CAD build for the part. Positions are in the model's coordinates, mm. A direction names the side the tool comes from. Give positions to 0.01 mm unless a question says otherwise; leave off trailing zeros. Order: outer loops, then holes, each group sorted by start corner. A loop starts at its lowest first (then second) coordinate and runs counter-clockwise, first axis right, second up.
Item 1: Band-saw the part on A-A on z = 86. Give the cut face in (x, y).
Item 2: Which spindle directions (+Z, -Z, +X, -X, +Y, -Y) get a long thin tool onto all of the face, cutting with end or side? Do faces 1 (the cylindrical face through (88.898, -0.022, 86.994)), 2 (the cylindrical face through (74.73, -0.02, 131.56)). Say none if no direction does.
Item 3: Band-saw the part on C-C on y = 0.65. Count the separate pieces of the cut face and the enclosed holes in it, plus the area to 3 significant figures.
Item 4: Wall check: L1, parallel to X at y = 0.05, z = 3.81; L2, parallel to Z at x = 11, y = 0.35; L3, parallel to Z at x = -45, y = 0.3. Give the ranges that are in metal, low to high.
Item 5: Two-plate mould, pull along X, no slides. Class faces 3 (the cylindrical face through (-25.4, 0, 118.8)), 4 (the flat face through (2, -1.588, 15)), 5 (the cylindrical face through (0.3, 0, 163.4)): released by +X, released by -X, zero draft, split by the parting line, or undercut.
Item 6: Band-saw the part on B-B on x = -84. Give the cut face in (y, z).
Item 7: Flat gauge pin, fed straight in: P1, Ø1, axis at x = -34, y = 1.5, coming from the +Z side. Where does the tip first touch, or does it go through?
Autodesk Inventor part; units mm, degrees
ref_plane "YZ Plane" through (0, 0, 0) normal (1, 0, 0) x (0, 1, 0)
ref_plane "XZ Plane" through (0, 0, 0) normal (0, 1, 0) x (-1, 0, 0)
ref_plane "XY Plane" through (0, 0, 0) normal (0, 0, 1) x (1, 0, 0)
sketch "Sketch1" plane through (0, 0, 0) normal (0, 1, 0) x (-1, 0, 0)
  line L0 (127, -82.55) -> (-127, -82.55)
  line L1 (-127, -82.55) -> (-127, 82.55)
  line L2 (127, 82.55) -> (127, -82.55)
  circle A0 centre (0, 150.7034) radius 6.35
  arc A1 (12.7, 150.7034) -> (-12.7, 150.7034) centre (0, 150.7034) ccw
  line L3 (79.375, 87.2034) -> (-79.375, 87.2034) construction
  line L4 (79.375, 96.7284) -> (-79.375, 96.7284)
  line L5 (-79.375, 77.6784) -> (79.375, 77.6784)
  arc A2 (79.375, 77.6784) -> (79.375, 96.7284) centre (79.375, 87.2034) ccw
  arc A3 (-79.375, 96.7284) -> (-79.375, 77.6784) centre (-79.375, 87.2034) ccw
  line L6 (94.1705, 96.449) -> (49.3141, 96.449)
  circle A4 centre (80.3783, 87.2034) radius 3.175
  circle A5 centre (63.1063, 87.2034) radius 3.175
  circle A6 centre (32.3469, 87.2034) radius 3.175
  circle A7 centre (15.0749, 87.2034) radius 3.175
  circle A8 centre (-15.6845, 87.2034) radius 3.175
  circle A9 centre (-32.9565, 87.2034) radius 3.175
  circle A10 centre (-63.7159, 87.2034) radius 3.175
  circle A11 centre (-80.9879, 87.2034) radius 3.175
  arc A12 (127, 82.55) -> (12.7, 150.7034) centre (0, -0.5186) ccw
  arc A13 (-12.7, 150.7034) -> (-127, 82.55) centre (0, -0.5186) ccw
  point P0 (0, 0)
  point P1 (127, 0)
  point P2 (0, -82.55)
  point P3 (0, 87.2034)
  point P4 (0, 87.2034)
  dimension "d0" = 12.7
  dimension "d1" = 6.35
  dimension "d4" = 254
  dimension "d5" = 19.05
  dimension "d6" = 177.8
  dimension "d10" = 63.5
  dimension "d15" = 165.1
extrude "Extrusion1" add sketch "Sketch1" along normal mid plane 3.175 contours L0 L1 A13 A1 A12 L2
sketch "Sketch2" plane through (0, 1.5875, 0) normal (0, 1, 0) x (1, 0, 0)
  line L0 (-49.3141, -31.933) -> (-94.1705, -31.933)
  line L1 (-94.1705, -31.933) -> (-94.1705, -96.449)
  line L2 (-94.1705, -96.449) -> (-49.3141, -96.449)
  line L3 (-49.3141, -96.449) -> (-49.3141, -31.933)
  circle A0 centre (-53.5813, -71.049) radius 1.5875
  circle A1 centre (-89.9033, -71.049) radius 1.5875
  line L4 (-1.2827, -31.933) -> (-46.1391, -31.933)
  line L5 (-46.1391, -31.933) -> (-46.1391, -96.449)
  line L6 (-46.1391, -96.449) -> (-1.2827, -96.449)
  line L7 (-1.2827, -96.449) -> (-1.2827, -31.933)
  circle A2 centre (-5.5499, -71.049) radius 1.5875
  circle A3 centre (-41.8719, -71.049) radius 1.5875
  line L8 (46.7487, -31.933) -> (1.8923, -31.933)
  line L9 (1.8923, -31.933) -> (1.8923, -96.449)
  line L10 (1.8923, -96.449) -> (46.7487, -96.449)
  line L11 (46.7487, -96.449) -> (46.7487, -31.933)
  circle A4 centre (42.4815, -71.049) radius 1.5875
  circle A5 centre (6.1595, -71.049) radius 1.5875
  line L12 (94.7801, -31.933) -> (49.9237, -31.933)
  line L13 (49.9237, -31.933) -> (49.9237, -96.449)
  line L14 (49.9237, -96.449) -> (94.7801, -96.449)
  line L15 (94.7801, -96.449) -> (94.7801, -31.933)
  circle A6 centre (90.5129, -71.049) radius 1.5875
  circle A7 centre (54.1909, -71.049) radius 1.5875
  circle A8 centre (-68.834, 3.81) radius 1.5875
  circle A9 centre (-54.6269, 54.61) radius 1.5875
  circle A10 centre (-97.79, 3.81) radius 1.5875
  circle A11 centre (-102.87, 54.61) radius 1.5875
  line L16 (-61.3664, 81.9424) -> (-73.3552, 81.9424)
  line L17 (-73.3552, 81.9424) -> (-73.3552, 69.85)
  line L18 (-73.3552, 69.85) -> (-105.41, 69.85)
  line L19 (-105.41, 69.85) -> (-105.41, 1.27)
  line L20 (-105.41, 1.27) -> (-52.324, 1.27)
  line L21 (-52.324, 1.27) -> (-52.324, 69.85)
  line L22 (-52.324, 69.85) -> (-61.3664, 69.85)
  line L23 (-61.3664, 69.85) -> (-61.3664, 81.9424)
  line L24 (9.144, -5.08) -> (9.144, 69.85)
  line L25 (9.144, 69.85) -> (-45.974, 69.85)
  line L26 (-45.974, 69.85) -> (-45.974, -5.08)
  line L27 (-45.974, -5.08) -> (9.144, -5.08)
  circle A12 centre (-42.418, -1.524) radius 1.4605
  circle A13 centre (5.588, -1.524) radius 1.4605
  circle A14 centre (5.588, 66.294) radius 1.4605
  circle A15 centre (-42.418, 66.294) radius 1.4605
  line L28 (78.994, -6.985) -> (78.994, 69.85)
  line L29 (78.994, 69.85) -> (28.194, 69.85)
  line L30 (28.194, 69.85) -> (28.194, -6.985)
  line L31 (28.194, -6.985) -> (78.994, -6.985)
  circle A16 centre (75.819, -3.81) radius 1.5875
  circle A17 centre (75.819, 66.675) radius 1.5875
  circle A18 centre (31.369, 66.675) radius 1.5875
  circle A19 centre (31.369, -3.81) radius 1.5875
  circle A20 centre (-102.87, 54.61) radius 1.5875
  circle A21 centre (-54.6269, 54.61) radius 1.5875
  circle A22 centre (-68.834, 3.81) radius 1.5875
  circle A23 centre (-97.79, 3.81) radius 1.5875
  circle A24 centre (-42.418, 66.294) radius 1.5875
  circle A25 centre (-42.418, -1.524) radius 1.5875
  circle A26 centre (5.588, -1.524) radius 1.5875
  circle A27 centre (5.588, 66.294) radius 1.5875
  circle A28 centre (31.369, 66.675) radius 1.5875
  circle A29 centre (75.819, 66.675) radius 1.5875
  circle A30 centre (75.819, -3.81) radius 1.5875
  circle A31 centre (31.369, -3.81) radius 1.5875
  circle A32 centre (90.5129, -71.049) radius 1.5875
  circle A33 centre (54.1909, -71.049) radius 1.5875
  circle A34 centre (42.4815, -71.049) radius 1.5875
  circle A35 centre (6.1595, -71.049) radius 1.5875
  circle A36 centre (-5.5499, -71.049) radius 1.5875
  circle A37 centre (-41.8719, -71.049) radius 1.5875
  circle A38 centre (-53.5813, -71.049) radius 1.5875
  circle A39 centre (-89.9033, -71.049) radius 1.5875
  point P0 (0, 0)
extrude "Extrusion2" cut sketch "Sketch2" against normal through all contours A0 | A1 | A2 | A3 | A4 | A5 | A6 | A7 | A8 | A9 | A10 | A11 | A12 | A13 | A14 | A15 | A16 | A17 | A18 | A19 | A24 | A27
fillet "Fillet1" radius 25.4 2 edges at (127, 0, 82.55) (-127, 0, 82.55)
sketch "Sketch3" plane through (0, 1.5875, 0) normal (0, 1, 0) x (1, 0, 0)
  arc A0 (-127, -74.6004) -> (-122.0238, -89.701) centre (-101.6, -74.6004) ccw
  arc A1 (-122.0238, -89.701) -> (-12.7, -150.7034) centre (0, 0.5186) ccw
  arc A2 (-12.7, -150.7034) -> (12.7, -150.7034) centre (0, -150.7034) ccw
  arc A3 (12.7, -150.7034) -> (122.0238, -89.701) centre (0, 0.5186) ccw
  arc A4 (122.0238, -89.701) -> (127, -74.6004) centre (101.6, -74.6004) ccw
  line L0 (127, -74.6004) -> (127, 82.55)
  line L1 (127, 82.55) -> (-127, 82.55)
  line L2 (-127, 82.55) -> (-127, -74.6004)
  circle A5 centre (-53.5813, -71.049) radius 1.5875
  circle A6 centre (54.1909, -71.049) radius 1.5875
  circle A7 centre (31.369, 66.675) radius 1.5875
  circle A8 centre (-42.418, -1.524) radius 1.4605
  circle A9 centre (-97.79, 3.81) radius 1.5875
  circle A10 centre (-68.834, 3.81) radius 1.5875
  circle A11 centre (5.588, -1.524) radius 1.4605
  circle A12 centre (31.369, -3.81) radius 1.5875
  circle A13 centre (42.4815, -71.049) radius 1.5875
  circle A14 centre (-5.5499, -71.049) radius 1.5875
  circle A15 centre (-89.9033, -71.049) radius 1.5875
  circle A16 centre (90.5129, -71.049) radius 1.5875
  circle A17 centre (75.819, 66.675) radius 1.5875
  circle A18 centre (-42.418, 66.294) radius 1.5875
  circle A19 centre (-102.87, 54.61) radius 1.5875
  circle A20 centre (-54.6269, 54.61) radius 1.5875
  circle A21 centre (5.588, 66.294) radius 1.5875
  circle A22 centre (75.819, -3.81) radius 1.5875
  circle A23 centre (6.1595, -71.049) radius 1.5875
  circle A24 centre (-41.8719, -71.049) radius 1.5875
  line L3 (79.375, -96.7284) -> (-79.375, -96.7284)
  arc A25 (-79.375, -77.6784) -> (-79.375, -96.7284) centre (-79.375, -87.2034) ccw
  line L4 (-79.375, -77.6784) -> (79.375, -77.6784)
  arc A26 (79.375, -96.7284) -> (79.375, -77.6784) centre (79.375, -87.2034) ccw
  circle A27 centre (0, -150.7034) radius 6.35
  line L5 (-25.4, -118.9534) -> (25.4, -118.9534) construction
  line L6 (-19.05, -125.3034) -> (19.05, -125.3034)
  line L7 (19.05, -112.6034) -> (-19.05, -112.6034)
  arc A28 (-19.05, -112.6034) -> (-19.05, -125.3034) centre (-19.05, -118.9534) ccw
  arc A29 (19.05, -125.3034) -> (19.05, -112.6034) centre (19.05, -118.9534) ccw
  point P0 (0, 0)
  point P1 (0, -118.9534)
  dimension "d17" = 50.8
  dimension "d18" = 12.7
  dimension "d19" = 25.4
extrude "Extrusion3" cut sketch "Sketch3" against normal blind 3.175 contours A28 L7 A29 L6
properties part number "Top Plate"
The answers:
1. outline: (-124.3, -1.59) - (-88.82, -1.59) - (-88.82, 1.59) - (-124.3, 1.59) - close; (88.82, -1.59) - (124.3, -1.59) - (124.3, 1.59) - (88.82, 1.59) - close
2. face 1: +Y, -Y
2. face 2: +Z, +X, +Y, -Y
3. separate pieces: 1
3. enclosed holes: 23
3. area: 50,200 mm2
4. L1: x = -127 to 29.78, 32.96 to 74.23, 77.41 to 127
4. L2: z = -82.55 to 77.68, 96.73 to 112.6, 125.3 to 157.05
4. L3: z = -82.55 to 77.68, 96.73 to 144.41
5. face 3: undercut
5. face 4: zero draft
5. face 5: split by the parting line
6. outline: (-1.59, -82.55) - (1.59, -82.55) - (1.59, 78.88) - (-1.59, 78.88) - close; (-1.59, 95.53) - (1.59, 95.53) - (1.59, 125.87) - (-1.59, 125.87) - close
7. P1: stops at z = 147.49
